Input: part model. Units: mm. Frame: model coordinates. Give positions to 0.01 mm unless a question says otherwise; leave off trailing zeros. Loops run counter-clockwise (first coordinate to the right, second up) from the corner with the lowest first, then second, coordinate; pieces in that order, holes last. Notation, with made-up numbers: (-33, 78.25) - (-25, 78.25) arc R10 ccw to (-25, 97.25) - close; hole circle Ø10 at (7.5, 6). An arc over 180 degrees is marked (long way). Answer as a JSON object with one key per item and string values. Group by question number.
(1) Pin query (flat end, axial travel): P1, Ø1, axis at y = -67, z = -3, coming from the -X side; P2, Ø2.5, axis at x = 100, z = -2, coming from the +Y side; P3, Ø1.5, axis at x = 127, y = -50.5, coming from the +Z side; P4, Ø1.6, axis at y = -22, z = 1.5, coming from the -X side. Return the tip coordinate at first contact, or that it passes through.
(2) Section query A-A (y = -50.5). Return loops of the section in (x, z).
(3) Section query D-D (x = 94). Count the separate pieces of the cut face and the enclosed holes in it, plus the area to 3 significant figures.
(4) Material intervals for L1, parallel to X at y = -85, z = -0.25; L2, parallel to X at y = -16.5, z = -0.25; L3, parallel to Y at x = 117.5, z = -2.4, sorted ascending.
```python
from build123d import *

# Parameters (mm, degrees)
F0_W     = 145
F0_H     = 95
F0_R     = 1.5
F0_W_2   = 12
F0_H_2   = 12
F0_W_3   = 105
F0_H_3   = 17
F1_DEPTH = 5
F3_DEPTH = 2
F5_DEPTH = 200


with BuildPart() as f1:
    # F0 (on Top) → F1 (new body)
    with BuildSketch(Plane.XY):
        with Locations((72.5, -47.5)):
            Rectangle(F0_W, F0_H)
        with Locations((27.5, -76.787904)):
            Circle(F0_R, mode=Mode.SUBTRACT)
        with Locations((47, -80)):
            Rectangle(F0_W_2, F0_H_2, mode=Mode.SUBTRACT)
        with Locations((64, -80)):
            Rectangle(F0_W_2, F0_H_2, mode=Mode.SUBTRACT)
        with Locations((47, -63)):
            Rectangle(F0_W_2, F0_H_2, mode=Mode.SUBTRACT)
        with Locations((64, -63)):
            Rectangle(F0_W_2, F0_H_2, mode=Mode.SUBTRACT)
        with Locations((81, -80)):
            Rectangle(F0_W_2, F0_H_2, mode=Mode.SUBTRACT)
        with Locations((98, -80)):
            Rectangle(F0_W_2, F0_H_2, mode=Mode.SUBTRACT)
        with Locations((117.5, -76.787904)):
            Circle(F0_R, mode=Mode.SUBTRACT)
        with Locations((81, -63)):
            Rectangle(F0_W_2, F0_H_2, mode=Mode.SUBTRACT)
        with Locations((98, -63)):
            Rectangle(F0_W_2, F0_H_2, mode=Mode.SUBTRACT)
        with Locations((47, -46)):
            Rectangle(F0_W_2, F0_H_2, mode=Mode.SUBTRACT)
        with Locations((64, -46)):
            Rectangle(F0_W_2, F0_H_2, mode=Mode.SUBTRACT)
        with Locations((81, -46)):
            Rectangle(F0_W_2, F0_H_2, mode=Mode.SUBTRACT)
        with Locations((98, -46)):
            Rectangle(F0_W_2, F0_H_2, mode=Mode.SUBTRACT)
        with Locations((72.5, -21.5)):
            Rectangle(F0_W_3, F0_H_3, mode=Mode.SUBTRACT)
    extrude(amount=-F1_DEPTH)

    # F2 (on Top) → F3 (join)
    with BuildSketch(Plane.XY):
        with BuildLine():
            Line((129, 0), (11, 0))
            Line((11, 0), (11, -34))
            ThreePointArc((11, -34), (11.292893, -34.707107), (12, -35))
            Line((12, -35), (130.863056, -35))
            ThreePointArc((130.863056, -35), (131.570163, -34.707107), (131.863056, -34))
            Line((131.863056, -34), (131.863056, -21.256752))
            ThreePointArc((131.863056, -21.256752), (131.699365, -20.464306), (131.235085, -19.801577))
            Line((131.235085, -19.801577), (129.627971, -18.286291))
            ThreePointArc((129.627971, -18.286291), (129.163691, -17.623561), (129, -16.831115))
            Line((129, -16.831115), (129, 0))
        make_face()
        with BuildLine():
            Line((20.000057, -28.999976), (20.000057, -12.999976))
            Line((20.000057, -12.999976), (125.000057, -12.999976))
            Line((125.000057, -12.999976), (125.000057, -28.999976))
            ThreePointArc((125.000057, -28.999976), (124.707164, -29.707083), (124.000057, -29.999976))
            Line((124.000057, -29.999976), (21.000057, -29.999976))
            ThreePointArc((21.000057, -29.999976), (20.292951, -29.707083), (20.000057, -28.999976))
        make_face(mode=Mode.SUBTRACT)
    extrude(amount=F3_DEPTH)

    # F4 (on face) → F5 (cut)
    with BuildSketch(Plane(origin=(0, 0, 0), x_dir=(0, -1, 0), z_dir=(-1, 0, 0))):
        Polygon((0, 5), (0, -5), (8.390996, 5), align=None)
    extrude(amount=-F5_DEPTH, mode=Mode.SUBTRACT)


solid = f1.part
```
Recorded:
{
 "1": {"P1": "stops at x = 0", "P2": "stops at y = -1.47", "P3": "stops at z = 0", "P4": "stops at x = 11"},
 "2": {"outline": "(0, -5) - (41, -5) - (41, 0) - (0, 0) - close; (53, -5) - (58, -5) - (58, 0) - (53, 0) - close; (70, -5) - (75, -5) - (75, 0) - (70, 0) - close; (87, -5) - (92, -5) - (92, 0) - (87, 0) - close; (104, -5) - (145, -5) - (145, 0) - (104, 0) - close"},
 "3": {"separate pieces": "5", "enclosed holes": "0", "area": "225 mm^2"},
 "4": {"L1": "x = 0 to 41, 53 to 58, 70 to 75, 87 to 92, 104 to 145", "L2": "x = 0 to 20, 125 to 145", "L3": "y = -95 to -78.29, -75.29 to -30, -13 to -2.18"}
}
